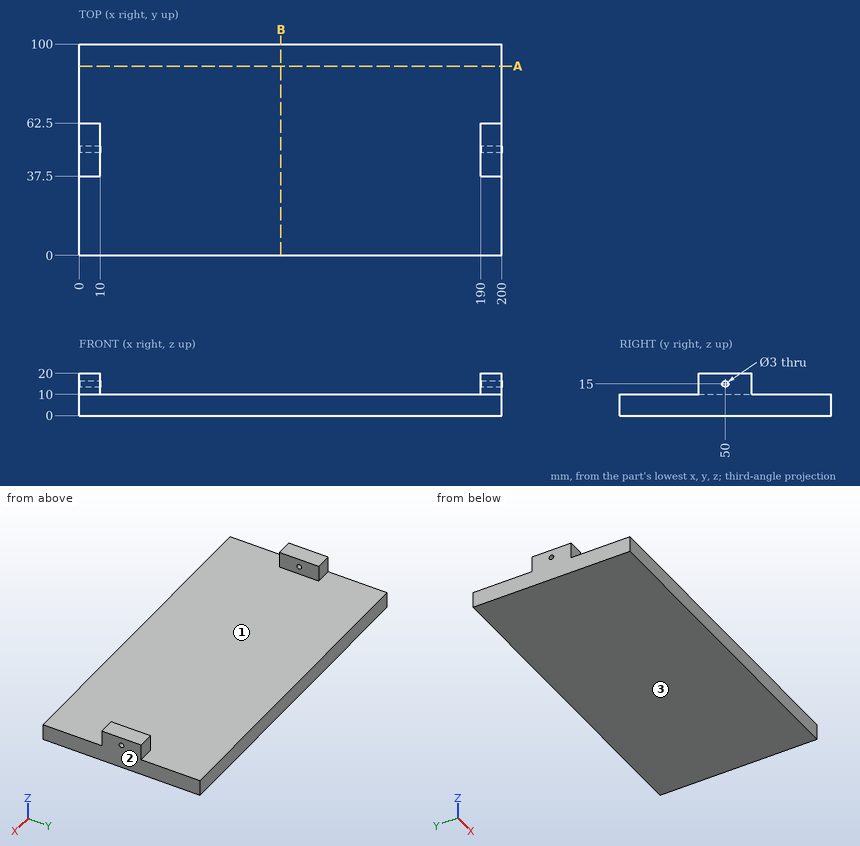
For this review, use the dimensioned drawing (mm, ordinates from the lowest corner) and the shaded views. Coordinates: 2 decimals unless noted, no trailing zeros. Loops run counter-clockwise (first coordinate to the right, second up) from the corner with the lowest first, then second, coordinate; pieces in that order, holes last. Notation, with made-up numbers: (23.5, -19) - (68.5, -19) arc R30 ccw to (68.5, 18) - close; hole circle Ø11 at (38.25, 5.5). An arc over 180 degrees is marked (long way). Use CSV: the item, a comma, the result in double quotes. Start each with the question number.
1) The part is to be moulded in two halves that separate along X. For the marked faces 1, 2 and 3, say which applies: +X half, -X half, draft (parallel to the pull), parting line (faces both ways), or undercut.
2) Wall thickness on L1, parallel to Y at x = 195.5, z = 15; L2, parallel to X at y = 50, z = 13.25; L3, parallel to Z at x = 161, y = 18.5: over which ranges is each line inside the solid? List them lowest first. Write a range as from..to.
3) For pin 1 Ø8 at (y, z) = (52.5, 13) entering from -X; pin 2 Ø8 at (x, z) = (4, 16) entering from +Y; pin 3 Ø5 at (x, z) = (2.5, 14) entering from -Y; pin 4 Ø1 at (x, y) = (123.5, 79.5) entering from +Z, all flat-tipped, find the tip position at first contact; note any pin that passes through.
4) Consider section A-A on y = 89.5. Write out the cut boundary in (x, z), then the cut area to 3 significant figures.
5) Consider section B-B on x = 95.5. Write out the cut boundary in (y, z).
Geometry says:
1,face 1,"undercut"
1,face 2,"+X half"
1,face 3,"draft"
2,L1,"37.5..48.5, 51.5..62.5"
2,L2,"0..10, 190..200"
2,L3,"0..10"
3,pin 1,"x = 0"
3,pin 2,"y = 62.5"
3,pin 3,"y = 37.5"
3,pin 4,"z = 10"
4,outline,"(0, 0) - (200, 0) - (200, 10) - (0, 10) - close"
4,area,"2,000 mm^2"
5,outline,"(0, 0) - (100, 0) - (100, 10) - (0, 10) - close"
